For this review, take the finished solid that the model builds, in its own axes (mm). A direction names the side the tool comes from. Coordinates: 2 decimals unless noted, no trailing zeros. Loops run counter-clockwise (first coordinate to the right, second up) from the corner with the lowest first, then second, coordinate; pieces in that order, holes last.
1. Take a section at B-B, the plane z = -2.5. State the section outline as (x, y) points, then the cut area to 3 significant figures.
2. Take a section at C-C, the plane z = -11. State the section outline as (x, y) points, then the cut area to 3 significant figures.
3. Clearance check with flat-ended pins moving along their axes: P1, Ø2.5, axis at x = -44.5, y = -6.08, coming from the -Z side; P2, Ø2, axis at y = -4.5, z = 4, coming from the -X side; P3, Ø5, axis at x = 38, z = -10, coming from the -Y side; P4, Ø2.5, axis at x = -45.5, y = -8.5, coming from the +Z side. State where each tip first meets the part, or that it passes through.
4. To check wall thickness, follow probe 1 along X at (y, z) = (0.3, 5); probe 2 along X at (y, z) = (0.75, 8.25); probe 3 along Y at (x, z) = (-44.5, 5.85). State the ranges of each line that lie inside material, in increasing order.
5. Take a section at A-A, the plane x = -44.5. State the section outline as (y, z) points.
6. Mouldability with a two-part tool opening along X and no side actions: class faces 6 (the face through (50, -2.8, 3.8)), 7 (the face through (-59.82, 0.79, 4.55)), 8 (the face through (45, -11.54, 7)) as pulls with the +X half, pulls with the -X half, needs draft (parallel to the pull), parting line crosses it, or undercut.
7. Machinability: for faces 1 (the face through (-46, -11.54, 7)), 2 (the face through (28, 0, 8.5)), 3 (the face through (45, -8, 8.5)), 4 (the face through (-46, -8, 4.5)), 5 (the face through (41, -7, 6)), which of the approach directions +Z, -Z, +X, -X, +Y, -Y give a long, thin tool a straight path to every point of the face, cutting with its end or side? Answer none if there is none.
8. Take a section at D-D, the plane x = 61.25. State the section outline as (y, z) points, then the cut area to 3 significant figures.
```python
from build123d import *

# Parameters (mm, degrees)
SKETCH1_W           = 128.6
SKETCH1_H           = 25
SKETCH1_R           = 1.5
SKETCH1_W_2         = 17.508
SKETCH1_H_2         = 14.090792215
BOSS_EXTRUDE1_DEPTH = 1.6
SKETCH3_W           = 100
SKETCH3_H           = 25
SKETCH3_W_2         = 17.508
SKETCH3_H_2         = 14.090792215
BOSS_EXTRUDE4_DEPTH = 2.54
SKETCH4_W           = 9
SKETCH4_H           = 9
SKETCH4_R           = 1.5
BOSS_EXTRUDE5_DEPTH = 4
FILLET1_R           = 2


with BuildPart() as part:
    # Sketch1 → Boss-Extrude1 (new body)
    with BuildSketch(Plane(origin=(0, 0, 0), x_dir=(1, 0, 0), z_dir=(0, 1, 0))):
        Rectangle(SKETCH1_W, SKETCH1_H)
        with Locations((-61.25, -5)):
            Circle(SKETCH1_R, mode=Mode.SUBTRACT)
        with Locations((61.25, -5)):
            Circle(SKETCH1_R, mode=Mode.SUBTRACT)
        with Locations((28.271706015, -1.454603892)):
            Rectangle(SKETCH1_W_2, SKETCH1_H_2, mode=Mode.SUBTRACT)
    extrude(amount=BOSS_EXTRUDE1_DEPTH)

    # Sketch3 → Boss-Extrude4 (add)
    with BuildSketch(Plane(origin=(0, 0, 0), x_dir=(1, 0, 0), z_dir=(0, 1, 0))):
        Rectangle(SKETCH3_W, SKETCH3_H)
        with Locations((28.271706015, -1.454603892)):
            Rectangle(SKETCH3_W_2, SKETCH3_H_2, mode=Mode.SUBTRACT)
    extrude(amount=-BOSS_EXTRUDE4_DEPTH)

    # Sketch4 → Boss-Extrude5 (add)
    with BuildSketch(Plane.XY.offset(8.5)):
        with Locations((-45.5, -7.04)):
            Rectangle(SKETCH4_W, SKETCH4_H)
        with Locations((-44.5, -6.08)):
            Circle(SKETCH4_R, mode=Mode.SUBTRACT)
        with Locations((45.5, -7.04)):
            Rectangle(SKETCH4_W, SKETCH4_H)
        with Locations((44.5, -6.08)):
            Circle(SKETCH4_R, mode=Mode.SUBTRACT)
    extrude(amount=-BOSS_EXTRUDE5_DEPTH)

    # Fillet1
    fillet1_edges = [part.edges().sort_by_distance(p)[0] for p in [
        (-45.5, -2.54, 4.5),
        (45.5, -2.54, 4.5),
    ]]
    fillet(fillet1_edges, radius=FILLET1_R)


solid = part.part
```
Results list:
1. outline: (-64.3, 0) - (-50, 0) - (-50, -2.54) - (19.52, -2.54) - (19.52, 1.6) - (-64.3, 1.6) - close; (37.03, -2.54) - (50, -2.54) - (50, 0) - (64.3, 0) - (64.3, 1.6) - (37.03, 1.6) - close
1. area: 387 mm2
2. outline: (-64.3, 0) - (-50, 0) - (-50, -2.54) - (50, -2.54) - (50, 0) - (64.3, 0) - (64.3, 1.6) - (-64.3, 1.6) - close
2. area: 460 mm2
3. P1: passes through
3. P2: stops at x = -50
3. P3: stops at y = -2.54
3. P4: stops at z = 8.5
4. probe 1: x = -64.3 to -62.75, -59.75 to 19.52, 37.03 to 59.75, 62.75 to 64.3
4. probe 2: x = -64.3 to 19.52, 37.03 to 64.3
4. probe 3: y = -11.54 to -7.58, -4.58 to 1.6
5. outline: (-11.54, 4.5) - (-7.58, 4.5) - (-7.58, 8.5) - (-11.54, 8.5) - close; (-4.58, 4.5) - (-4.54, 4.5) arc R2 cw to (-2.54, 2.5) - (-2.54, -12.5) - (1.6, -12.5) - (1.6, 12.5) - (-2.54, 12.5) - (-2.54, 8.5) - (-4.58, 8.5) - close
6. face 6: pulls with the +X half
6. face 7: undercut
6. face 8: needs draft
7. face 1: +Z, -Z, +X, -X, -Y
7. face 2: +Y, -Y
7. face 3: +Z, +X, -X, -Y
7. face 4: -Z, +X, -X, -Y
7. face 5: +Z, -Z, -Y
8. outline: (0, -12.5) - (1.6, -12.5) - (1.6, 3.5) - (0, 3.5) - close; (0, 6.5) - (1.6, 6.5) - (1.6, 12.5) - (0, 12.5) - close
8. area: 35.2 mm2
